from build123d import *

# Parameters (mm, degrees)
SKETCH_R    = 1.5
SKETCH001_R = 1.5
SKETCH002_R = 2.5
SKETCH003_R = 2.5
SKETCH004_R = 1.5
SKETCH005_R = 1.5
SKETCH006_R = 0.575
PAD_DEPTH   = 3


with BuildPart() as part:
    # Sketch → AdditiveLoft section 0
    with BuildSketch(Plane.XY):
        Circle(SKETCH_R)
    # Sketch001 (on DatumPlane) → AdditiveLoft section 1
    with BuildSketch(Plane.XY.offset(2)):
        Circle(SKETCH001_R)
    # Sketch002 (on DatumPlane) → AdditiveLoft section 2
    with BuildSketch(Plane(origin=(0, 0, 3), x_dir=(0, 1, 0), z_dir=(0, 0, 1))):
        Circle(SKETCH002_R)
    # Sketch003 (on DatumPlane) → AdditiveLoft section 3
    with BuildSketch(Plane(origin=(0, 0, 26), x_dir=(0, 1, 0), z_dir=(0, 0, 1))):
        Circle(SKETCH003_R)
    # Sketch004 (on DatumPlane) → AdditiveLoft section 4
    with BuildSketch(Plane(origin=(0, 0, 27), x_dir=(-1, 0, 0), z_dir=(0, 0, 1))):
        Circle(SKETCH004_R)
    # Sketch005 (on DatumPlane) → AdditiveLoft section 5
    with BuildSketch(Plane(origin=(0, 0, 57), x_dir=(0, -1, 0), z_dir=(0, 0, 1))):
        Circle(SKETCH005_R)
    loft(ruled=True)

    # Sketch006 (on Face1 of AdditiveLoft) → Pad (new body)
    with BuildSketch(Plane(origin=(0, 0, 0), x_dir=(1, 0, 0), z_dir=(0, 0, -1))):
        Circle(SKETCH006_R)
    extrude(amount=PAD_DEPTH)


solid = part.part
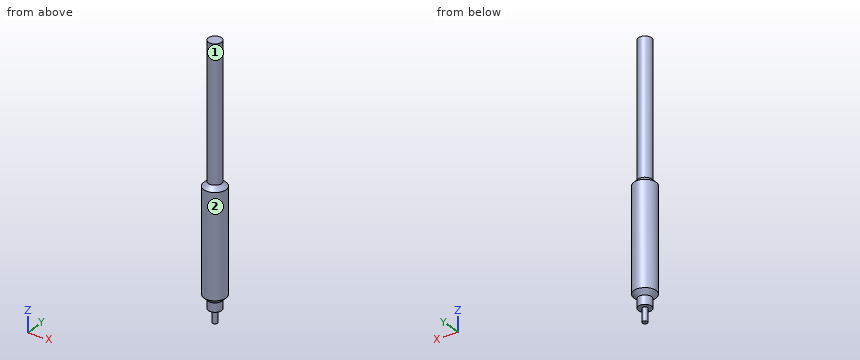
Part model, mm, in its own coordinate system. Face numbers are marked on the shaded views. A direction names the side the tool comes from. Round coordinates to 2 decimals unless told otherwise and drop trailing zeros. Write each loop counter-clockwise with the first axis right and the second up, starting at its lowest first coordinate (ties: lowest second). Pieces come first, ordered by that corner, then holes. Notation, with made-up numbers: M 48,6 L 96,6 A30 ccw 96,45 Z; hole C 45,-27.5 d10. An arc over 180 degrees is marked long. Return JSON: item names as keys, results as strings. Group by question number.
(1) Pin check, flat tips, straight feed: pin 1 Ø1.5 at (x, z) = (0.5, 23.5) entering from -Y; pin 2 Ø2 at (x, y) = (2, 0.5) entering from -Z; pin 3 Ø3 at (x, z) = (-2, 48.5) entering from +Y; pin 4 Ø2 at (y, z) = (1.5, 19.5) entering from -X. Stop position of each tip, or through.
(2) Drill centre lines: probe 1 along Y at (x, z) = (0.15, 1.5); probe 2 along Z at (x, y) = (-0.5, -1.95); probe 3 along X at (y, z) = (-0.2, 19). Where is each one in solid material? Low to high.
(3) Saw through at A-A on z = 29. Write the cut outline in (x, y), then the cut area to 3 significant figures.
(4) Saw through at B-B on z = 2.5. Write the cut outline in (x, y), then the cut area to 3 significant figures.
(5) Which spindle directions (+Z, -Z, +X, -X, +Y, -Y) get a long thin tool onto all of the face, cutting with end or side? Do the marked faces 1 and 2. Say none if no direction does.
Returned:
{
 "1": {"pin 1": "y = -2.5", "pin 2": "z = 0", "pin 3": "y = 1.41", "pin 4": "x = -2.45"},
 "2": {"probe 1": "-1.49 to 1.49", "probe 2": "2.51 to 26.49", "probe 3": "-2.49 to 2.49"},
 "3": {"outline": "C 0,0 d3", "area": "7.07 mm²"},
 "4": {"outline": "C 0,0 d4", "area": "12.6 mm²"},
 "5": {"face 1": "+Z", "face 2": "+Z, -Z"}
}
